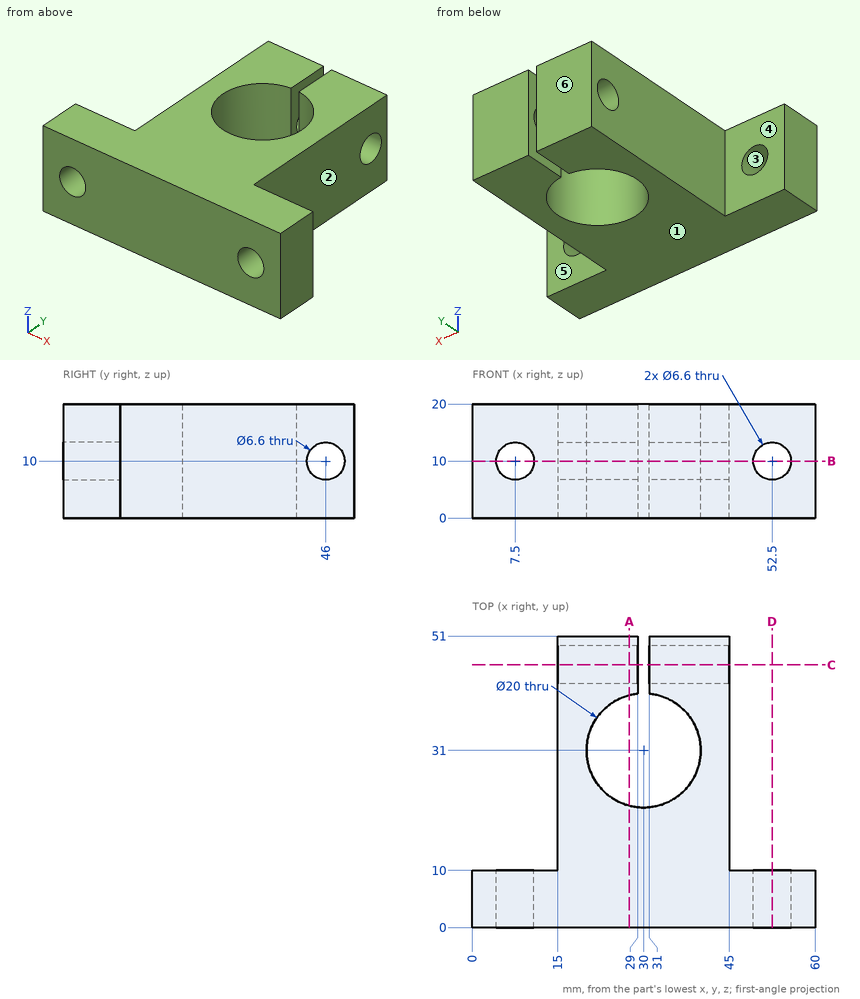
For this review, use the dimensioned drawing (mm, ordinates from the lowest corner) and the shaded views. A direction names the side the tool comes from. Round coordinates to 2 decimals unless told otherwise and drop trailing zeros. Write each loop counter-clockwise with the first axis right and the second up, starting at its lowest first coordinate (ties: lowest second). Pieces come first, ordered by that corner, then holes. Notation, with made-up numbers: (34, 4.25) - (51, 4.25) arc R21 cw to (51, 41.25) - close; hole circle Ø10 at (58.25, 16.5). An arc over 180 degrees is marked (long way). Use a Markdown table: item, result.
Q1. We need section A-A (x = 27.5). Give the boundary of the cut face in (y, z).
Derived:
| item | result |
|---|---|
| outline | (0, 0) - (21.32, 0) - (21.32, 20) - (0, 20) - close; (40.68, 0) - (51, 0) - (51, 20) - (40.68, 20) - close; hole circle Ø6.6 at (46, 10) |
Q2. Machinability: for the marked faces 4, 5 and 6, which of the approach directions +Z, -Z, +X, -X, +Y, -Y give a long, thin tool a straight path to every point of the face, cutting with its end or side? Answer none if there is none.
Derived:
| item | result |
|---|---|
| face 4 | +Z, -Z, -X, +Y |
| face 5 | +Z, -Z, +X, +Y |
| face 6 | +Z, -Z, +X, -X, +Y |
Q3. We need section B-B (z = 10). Give the boundary of the cut face in (x, y), plus the area to 3 significant figures.
Derived:
| item | result |
|---|---|
| outline | (0, 0) - (4.2, 0) - (4.2, 10) - (0, 10) - close; (10.8, 0) - (49.2, 0) - (49.2, 10) - (45, 10) - (45, 42.7) - (31, 42.7) - (31, 40.95) arc R10 cw (long way) to (29, 40.95) - (29, 42.7) - (15, 42.7) - (15, 10) - (10.8, 10) - close; (15, 49.3) - (29, 49.3) - (29, 51) - (15, 51) - close; (31, 49.3) - (45, 49.3) - (45, 51) - (31, 51) - close; (55.8, 0) - (60, 0) - (60, 10) - (55.8, 10) - close |
| area | 1,180 mm2 |
Q4. We need section C-C (y = 46). Give the boundary of the cut face in (x, z).
Derived:
| item | result |
|---|---|
| outline | (15, 0) - (29, 0) - (29, 6.7) - (15, 6.7) - close; (15, 13.3) - (29, 13.3) - (29, 20) - (15, 20) - close; (31, 0) - (45, 0) - (45, 6.7) - (31, 6.7) - close; (31, 13.3) - (45, 13.3) - (45, 20) - (31, 20) - close |
Q5. We need section D-D (x = 52.5). Give the boundary of the cut face in (y, z), plus the area to 3 significant figures.
Derived:
| item | result |
|---|---|
| outline | (0, 0) - (10, 0) - (10, 6.7) - (0, 6.7) - close; (0, 13.3) - (10, 13.3) - (10, 20) - (0, 20) - close |
| area | 134 mm2 |
Q6. Clearance check with flat-ended pins moving along their axes: pin 1 (10 mm diameter, centred on y = 20.5, z = 7.5, fed in from +X); pin 2 (5.5 mm diameter, centred on y = 46, z = 10, fed in from -X); pin 3 (10.5 mm diameter, centred on y = 46, z = 10, fed in from -X); pin 4 (5 mm diameter, centred on x = 53.5, z = 7.5, fed in from +Y). State where each tip first meets the part, or that it passes through.
Derived:
| item | result |
|---|---|
| pin 1 | stops at x = 45 |
| pin 2 | passes through |
| pin 3 | stops at x = 15 |
| pin 4 | stops at y = 10 |
Q7. The part is to be moulded in two halves that separate along Z. For the marked faces 1, 2 and 3, say which applies: pulls with the +Z half, pulls with the -Z half, needs draft (parallel to the pull), parting line crosses it, or undercut.
Derived:
| item | result |
|---|---|
| face 1 | pulls with the -Z half |
| face 2 | needs draft |
| face 3 | undercut |
Q8. Wall thickness on line 1 along X through (y, z) = (8.25, 10); line 2 along Y through (x, z) = (35, 10); line 3 along Y through (x, z) = (36.75, 10): over which ranges is each line inside the solid? List them lowest first.
Derived:
| item | result |
|---|---|
| line 1 | x = 0 to 4.2, 10.8 to 49.2, 55.8 to 60 |
| line 2 | y = 0 to 22.34, 39.66 to 42.7, 49.3 to 51 |
| line 3 | y = 0 to 23.62, 38.38 to 42.7, 49.3 to 51 |
